Could you check a few things on this model? Use its own coordinates, in mm. Face numbers are marked on the shaded views. Round coordinates to 2 decimals unless told otherwise and drop trailing zeros. Loops run counter-clockwise (first coordinate to the right, second up) from the corner with the lowest first, then second, coordinate; pieces in that order, holes last.
from build123d import *

# Parameters (mm, degrees)
BOSS_EXTRUDE1_DEPTH = 1.59
SKETCH2_W           = 1.59
SKETCH2_H           = 45
BOSS_EXTRUDE2_DEPTH = 30.41
SKETCH3_R           = 1.75
SKETCH3_R_2         = 2.5
CUT_EXTRUDE1_DEPTH  = 108.565311323
SKETCH4_R           = 2.5
SKETCH4_R_2         = 1.75
CUT_EXTRUDE2_DEPTH  = 30.41


with BuildPart() as part:
    # Sketch1 → Boss-Extrude1 (new body)
    with BuildSketch(Plane.XY):
        with BuildLine():
            Line((0, 14), (-98.41, 14))
            Line((-98.41, 14), (-98.41, -14))
            Line((-98.41, -14), (0, -14))
            ThreePointArc((0, -14), (14, 0), (0, 14))
        make_face()
    extrude(amount=BOSS_EXTRUDE1_DEPTH)

    # Sketch2 → Boss-Extrude2 (add)
    with BuildSketch(Plane(origin=(0, 0, 0), x_dir=(-1, 0, 0), z_dir=(0, 0, -1))):
        with Locations((97.615, -8.5)):
            Rectangle(SKETCH2_W, SKETCH2_H)
    extrude(amount=BOSS_EXTRUDE2_DEPTH)

    # Sketch3 → Cut-Extrude1 (cut, through all)
    with BuildSketch(Plane(origin=(0, 0, 0), x_dir=(-1, 0, 0), z_dir=(0, 0, -1))):
        with Locations((71.82, 0)):
            Circle(SKETCH3_R)
        with Locations((-8.5, 0)):
            Circle(SKETCH3_R)
        Circle(SKETCH3_R_2)
        with Locations((21.25, 0)):
            Circle(SKETCH3_R)
    extrude(amount=-CUT_EXTRUDE1_DEPTH, mode=Mode.SUBTRACT)

    # Sketch4 → Cut-Extrude2 (cut)
    with BuildSketch(Plane.ZY.offset(98.41)):
        with Locations((-15.205, 0)):
            Circle(SKETCH4_R)
        with Locations((-15.205, 8.5)):
            Circle(SKETCH4_R_2)
        with Locations((-15.205, -21.25)):
            Circle(SKETCH4_R_2)
    extrude(amount=-CUT_EXTRUDE2_DEPTH, mode=Mode.SUBTRACT)


solid = part.part
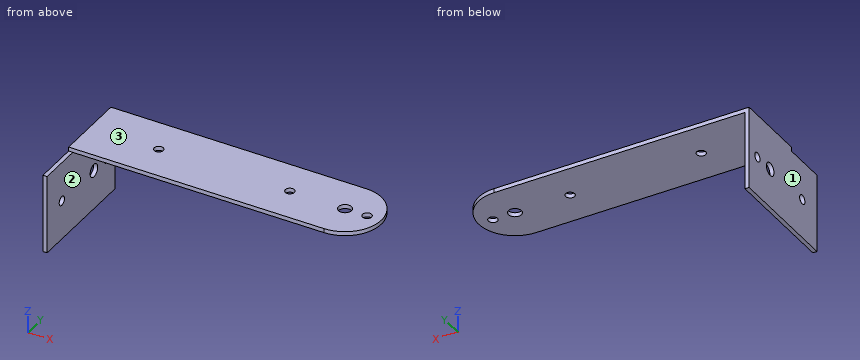
Item 1: We'd pull the mould along X, two halves only. Please class the marked faces 1, 2 and 3: released by +X, released by -X, zero draft, split by the parting line, or undercut.
Results list:
face 1: released by -X
face 2: released by +X
face 3: zero draft
Item 2: If we section it at D-D, the plane z = -23: Please give me the cut outline in (x, y), then the cut area to 4 significant figures.
Results list:
outline: (-98.41, -31) - (-96.82, -31) - (-96.82, 14) - (-98.41, 14) - close
area: 71.55 mm2
Item 3: If we section it at C-C, the plane y = 8.5: Please give me the cut outline in (x, z) (3 decimals).
Results list:
outline: (-98.41, -30.41) - (-96.82, -30.41) - (-96.82, -16.955) - (-98.41, -16.955) - close; (-98.41, -13.455) - (-96.82, -13.455) - (-96.82, 0) - (11.124, 0) - (11.124, 1.59) - (-98.41, 1.59) - close
Item 4: If we section it at B-B, the plane y = -21.25: Please give me the cut outline in (x, z) (3 decimals).
Results list:
outline: (-98.41, -30.41) - (-96.82, -30.41) - (-96.82, -16.955) - (-98.41, -16.955) - close; (-98.41, -13.455) - (-96.82, -13.455) - (-96.82, 0) - (-98.41, 0) - close
Item 5: If I drill on line 1 along Y through (x, z) = (-21.25, 0.65); line 2 along X through (y, z) = (-27, -1.5); line 3 along Z through (x, y) = (-13.5, 6), over which ranges is the centre line in solid material (lowest first)?
Results list:
line 1: y = -14 to -1.75, 1.75 to 14
line 2: x = -98.41 to -96.82
line 3: z = 0 to 1.59
Item 6: If we section it at A-A, the plane x = -71.82: Please give me the cut outline in (y, z).
Results list:
outline: (-14, 0) - (-1.75, 0) - (-1.75, 1.59) - (-14, 1.59) - close; (1.75, 0) - (14, 0) - (14, 1.59) - (1.75, 1.59) - close
Item 7: Will these pins go through, and if not, where does the flat tip stop? pin 1 (1.3 mm diameter, centred on x = -69, z = 0.5, fed in from -Y); pin 2 (5 mm diameter, centred on y = -4.5, z = -14.5, fed in from +X); pin 3 (1 mm diameter, centred on x = -32.5, y = 0, fed in from -Z).
Results list:
pin 1: stops at y = -14
pin 2: stops at x = -96.82
pin 3: stops at z = 0
